Part model, mm, in its own coordinate system. Face numbers are marked on the shaded views. A direction names the side the tool comes from. Coordinates: 2 decimals unless noted, no trailing zeros. Loops run counter-clockwise (first coordinate to the right, second up) from the corner with the lowest first, then second, coordinate; pieces in that order, holes last. Notation, with made-up numbers: (26, 8) - (30, 8) arc R20 ccw to (30, 46) - close; hole circle Ø1 at (41, -9). An arc over 180 degrees is marked (long way). Answer as CSV lines item,"result".
from build123d import *

# Parameters (mm, degrees)
SKETCH1_W           = 177.8
SKETCH1_H           = 254
BOSS_EXTRUDE1_DEPTH = 36.445
SHELL1_T            = 3
SKETCH2_R           = 22
CUT_EXTRUDE1_DEPTH  = 3
SKETCH3_R           = 5
SKETCH3_R_2         = 2.5
CUT_EXTRUDE2_DEPTH  = 3
SKETCH12_W          = 12
SKETCH12_H          = 66.89
BOSS_EXTRUDE5_DEPTH = 8
SKETCH10_R          = 3
CUT_EXTRUDE8_DEPTH  = 8
SKETCH13_W          = 174.8
SKETCH13_H          = 69.89
SKETCH13_W_2        = 171.8
SKETCH13_H_2        = 66.89
BOSS_EXTRUDE6_DEPTH = 25
SKETCH14_W          = 175.3
SKETCH14_H          = 70.39
SKETCH14_W_2        = 171.8
SKETCH14_H_2        = 66.89
CUT_EXTRUDE9_DEPTH  = 10
SKETCH17_W          = 171.8
SKETCH17_H          = 66.89
BOSS_EXTRUDE7_DEPTH = 2
SKETCH15_W          = 5
SKETCH15_H          = 5
CUT_EXTRUDE10_DEPTH = 5
BOSS_EXTRUDE8_DEPTH = 5


with BuildPart() as part:
    # Sketch1 → Boss-Extrude1 (new, symmetric)
    with BuildSketch(Plane.XY):
        Rectangle(SKETCH1_W, SKETCH1_H)
    extrude(amount=BOSS_EXTRUDE1_DEPTH, both=True)

    # Shell1 (no face opened: a closed hollow body)
    add(offset(amount=-SHELL1_T, mode=Mode.PRIVATE), mode=Mode.SUBTRACT)

    # Sketch2 → Cut-Extrude1 (cut)
    with BuildSketch(Plane(origin=(0, 0, 33.445), x_dir=(-1, 0, 0), z_dir=(0, 0, -1))):
        with Locations((0, -4)):
            Circle(SKETCH2_R)
    extrude(amount=-CUT_EXTRUDE1_DEPTH, mode=Mode.SUBTRACT)

    # Sketch3 → Cut-Extrude2 (cut)
    with BuildSketch(Plane.XY.offset(-33.445)):
        with Locations((24.1, -1)):
            Circle(SKETCH3_R)
        with Locations((44.229314747, 13.826013888)):
            Circle(SKETCH3_R_2)
        with Locations((38.926013888, 19.129314747)):
            Circle(SKETCH3_R_2)
        with Locations(Location((38.926013888, -21.129314747, 0), (0, 0, 180))):
            Circle(SKETCH3_R_2)
        with Locations(Location((44.229314747, -15.826013888, 0), (0, 0, 180))):
            Circle(SKETCH3_R_2)
        with Locations((0.36806178, 28.035239078)):
            Circle(SKETCH3_R_2)
        with Locations((-4.935239078, 22.73193822)):
            Circle(SKETCH3_R_2)
        with Locations(Location((-4.935239078, -24.73193822, 0), (0, 0, 180))):
            Circle(SKETCH3_R_2)
        with Locations(Location((0.36806178, -30.035239078, 0), (0, 0, 180))):
            Circle(SKETCH3_R_2)
        with Locations((16.6, -46)):
            Circle(SKETCH3_R_2)
        with Locations((16.6, -53.5)):
            Circle(SKETCH3_R_2)
    extrude(amount=-CUT_EXTRUDE2_DEPTH, mode=Mode.SUBTRACT)

    # Sketch12 → Boss-Extrude5 (add)
    with BuildSketch(Plane.XZ.offset(-124)):
        Rectangle(SKETCH12_W, SKETCH12_H)
    extrude(amount=BOSS_EXTRUDE5_DEPTH)

    # Sketch10 → Cut-Extrude8 (cut)
    with BuildSketch(Plane(origin=(0, 127, 0), x_dir=(1, 0, 0), z_dir=(0, 1, 0))):
        with Locations(Location((0, 0, 0), (0, 0, 270))):
            Circle(SKETCH10_R)
    extrude(amount=-CUT_EXTRUDE8_DEPTH, mode=Mode.SUBTRACT)


with BuildPart() as body_2:
    # Split2: the piece on the far side of the plane
    add(part.part)
    split(bisect_by=Plane.ZX.offset(52), keep=Keep.BOTTOM)

    # Sketch13 → Boss-Extrude6 (add)
    with BuildSketch(Plane(origin=(0, 52, 0), x_dir=(1, 0, 0), z_dir=(0, 1, 0))):
        Rectangle(SKETCH13_W, SKETCH13_H)
        Rectangle(SKETCH13_W_2, SKETCH13_H_2, mode=Mode.SUBTRACT)
    extrude(amount=BOSS_EXTRUDE6_DEPTH)

    # Sketch17 → Boss-Extrude7 (add)
    with BuildSketch(Plane(origin=(0, -124, 0), x_dir=(1, 0, 0), z_dir=(0, 1, 0))):
        Rectangle(SKETCH17_W, SKETCH17_H)
    extrude(amount=BOSS_EXTRUDE7_DEPTH)

    # Sketch15 → Cut-Extrude10 (cut)
    with BuildSketch(Plane.XZ.offset(127)):
        Polygon((11.604740411, 0), (5.802370205, 10.05), (-5.802370205, 10.05), (-11.604740411, 0), (-5.802370205, -10.05), (5.802370205, -10.05), align=None)
        with Locations((-17.67766953, 17.67766953)):
            Rectangle(SKETCH15_W, SKETCH15_H)
        with Locations((17.67766953, 17.67766953)):
            Rectangle(SKETCH15_W, SKETCH15_H)
        with Locations((17.67766953, -17.67766953)):
            Rectangle(SKETCH15_W, SKETCH15_H)
        with Locations((-17.67766953, -17.67766953)):
            Rectangle(SKETCH15_W, SKETCH15_H)
    extrude(amount=-CUT_EXTRUDE10_DEPTH, mode=Mode.SUBTRACT)


with BuildPart() as part_1:
    add(part.part)

    # Split2
    split(bisect_by=Plane.ZX.offset(52), keep=Keep.TOP)

    # Sketch14 → Cut-Extrude9 (cut)
    with BuildSketch(Plane.XZ.offset(-52)):
        Rectangle(SKETCH14_W, SKETCH14_H)
        Rectangle(SKETCH14_W_2, SKETCH14_H_2, mode=Mode.SUBTRACT)
    extrude(amount=-CUT_EXTRUDE9_DEPTH, mode=Mode.SUBTRACT)


with BuildPart() as body_3:
    # Split3: the piece on the far side of the plane
    add(body_2.part)
    split(bisect_by=Plane.XY, keep=Keep.BOTTOM)

    # Sketch19 → Boss-Extrude8 (add)
    with BuildSketch(Plane.XY):
        Polygon((-87.4, 77), (-85.9, 77), (-85.9, 75.5), (-85.9, -122), (-11.604740411, -122), (-11.604740411, -123.5), (-87.4, -123.5), align=None)
        Polygon((87.4, 77), (87.4, -123.5), (11.604740411, -123.5), (11.604740411, -122), (85.9, -122), (85.9, 75.5), (85.9, 77), align=None)
    extrude(amount=BOSS_EXTRUDE8_DEPTH)


with BuildPart() as body_2_1:
    add(body_2.part)

    # Split3
    split(bisect_by=Plane.XY, keep=Keep.TOP)


solid = body_3.part
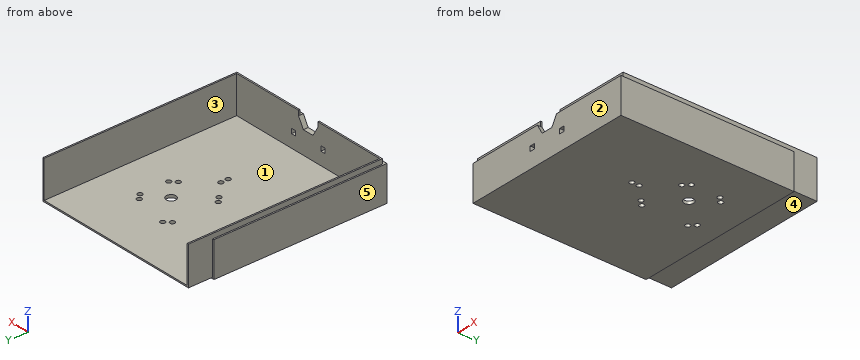
Q1. Two-plate mould, pull along X, no slides. Class the marked faces 3, 4 and 5: released by +X, released by -X, zero draft, split by the parting line, or undercut.
Results:
face 3,"undercut"
face 4,"zero draft"
face 5,"released by -X"
Q2. Saw through at A-A (y = -53.5). Give the cut face in (x, z) (3 decimals), then the cut area to 3 significant figures.
Results:
outline,"(-88.9, -36.445) - (14.1, -36.445) - (14.1, -33.445) - (-85.9, -33.445) - (-85.9, 5) - (-87.4, 5) - (-87.4, 0) - (-88.9, 0) - close; (19.1, -36.445) - (88.9, -36.445) - (88.9, 0) - (87.4, 0) - (87.4, 5) - (85.9, 5) - (85.9, -33.445) - (19.1, -33.445) - close"
area,"734 mm^2"
Q3. Which spindle directions (+Z, -Z, +X, -X, +Y, -Y) get a long thin tool onto all of the face, cutting with end or side? Do the marked faces 1 and 2. Say none if no direction does.
Results:
face 1,"+Z, +Y"
face 2,"+Z, -Z, +X, -X, -Y"
Q4. Saw through at D-D (z = -27.5). Give the cut face in (x, y), then the cut area to 3 significant figures.
Results:
outline,"(-88.9, -127) - (88.9, -127) - (88.9, 52) - (87.4, 52) - (87.4, 77) - (85.9, 77) - (85.9, -122) - (-85.9, -122) - (-85.9, 77) - (-87.4, 77) - (-87.4, 52) - (-88.9, 52) - close"
area,"2,010 mm^2"
Q5. Saw through at B-B (x = 24.1). Give the cut face in (y, z) (3 decimals).
Results:
outline,"(-127, -36.445) - (-6, -36.445) - (-6, -33.445) - (-122, -33.445) - (-122, 5) - (-123.5, 5) - (-123.5, 0) - (-127, 0) - close; (4, -36.445) - (52, -36.445) - (52, -34.945) - (77, -34.945) - (77, -33.445) - (4, -33.445) - close"
Q6. Flat gauge pins, fed straight in: pin 1 (10 mm diameter, centred on x = -44.5, y = -14.5, fed in from +Z) (3 decimals); pin 2 (1.2 mm diameter, centred on y = -122.5, z = 2, fed in from -X); pin 3 (10 mm diameter, centred on x = 18, z = -20, fed in from +Y). Where does each tip first touch, or does it go through?
Results:
pin 1,"stops at z = -33.445"
pin 2,"stops at x = -87.4"
pin 3,"stops at y = -122"
Q7. Saw through at C-C (x = -31). Give the cut face in (y, z) (3 decimals), then the cut area to 3 significant figures.
Results:
outline,"(-127, -36.445) - (52, -36.445) - (52, -34.945) - (77, -34.945) - (77, -33.445) - (-122, -33.445) - (-122, 5) - (-123.5, 5) - (-123.5, 0) - (-127, 0) - close"
area,"749 mm^2"
Q8. Wall check: L1, parallel to X at y = -46.5, z = -14; L2, parallel to Y at x = -24, z = -29; L3, parallel to X at y = 67, z = -7.5. Give the ranges that are in metal, low to high.
Results:
L1,"x = -88.9 to -85.9, 85.9 to 88.9"
L2,"y = -127 to -122"
L3,"x = -87.4 to -85.9, 85.9 to 87.4"
